Geometry check sheet. Reference: drawing and pictorial views, mm from the part's lowest x, y, z. Give positions to 0.01 mm unless a question says otherwise; leave off trailing zeros. Loops run counter-clockwise (first coordinate to the right, second up) from the corner with the lowest first, then second, coordinate; pieces in that order, holes last. Notation, with made-up numbers: (38, -39.5) - (43, -39.5) arc R32 cw to (43, -7.5) - close; hole circle Ø10 at (63, 19). An arc over 180 degrees is marked (long way). Use CSV: the item, a comma, the result in double quotes.
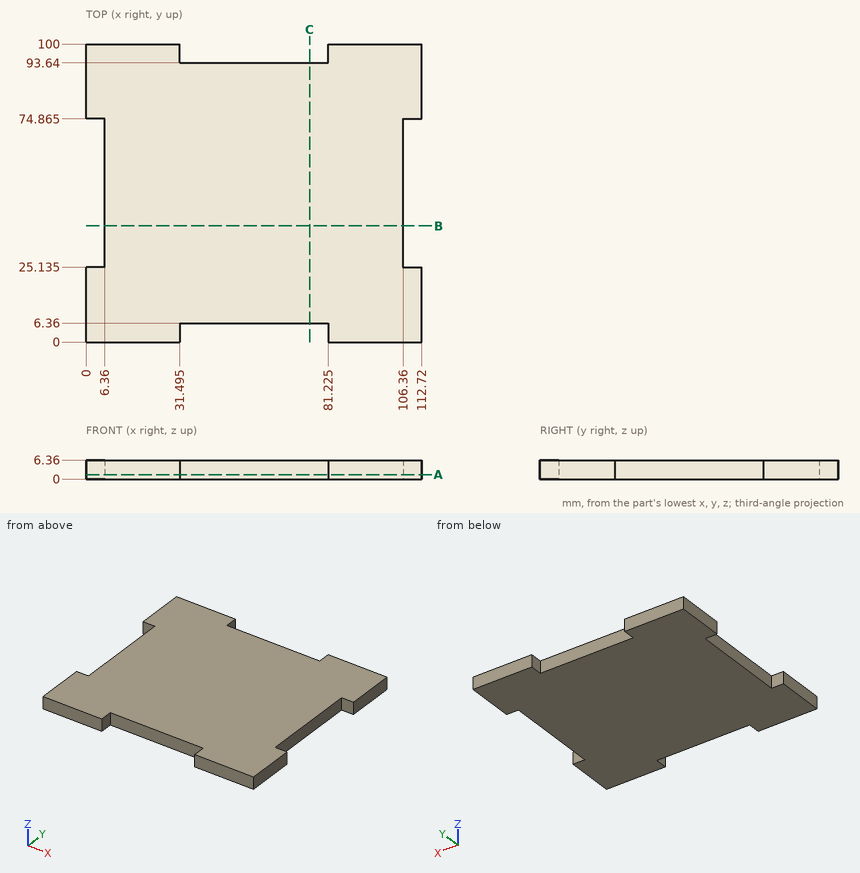
1. Go/stop test with flat-tipped pins: pin 1 Ø1.9 at (x, z) = (54, 2.5) entering from -Y; pin 2 Ø1.5 at (x, z) = (40.5, 5) entering from +Y; pin 3 Ø1.9 at (y, z) = (46.5, 2.5) entering from +X. Record where each tip stops, or that it passes through.
Completed:
pin 1,"stops at y = 6.36"
pin 2,"stops at y = 93.64"
pin 3,"stops at x = 106.36"
2. Sectioned sample at C-C, the plane x = 75. Record the boundary of the cut face in (y, z), and give its area (3 significant figures).
Completed:
outline,"(6.36, 0) - (93.64, 0) - (93.64, 6.36) - (6.36, 6.36) - close"
area,"555 mm²"
3. Sectioned sample at A-A, the plane z = 1.5. Record the boundary of the cut face in (x, y) (3 decimals).
Completed:
outline,"(0, 0) - (31.495, 0) - (31.495, 6.36) - (81.225, 6.36) - (81.225, 0) - (112.72, 0) - (112.72, 25.135) - (106.36, 25.135) - (106.36, 74.865) - (112.72, 74.865) - (112.72, 100) - (81.225, 100) - (81.225, 93.64) - (31.495, 93.64) - (31.495, 100) - (0, 100) - (0, 74.865) - (6.36, 74.865) - (6.36, 25.135) - (0, 25.135) - close"
4. Sectioned sample at B-B, the plane y = 39. Record the boundary of the cut face in (x, z).
Completed:
outline,"(6.36, 0) - (106.36, 0) - (106.36, 6.36) - (6.36, 6.36) - close"
5. Scan lines: line 1 along Y through (x, z) = (39, 4.75); line 2 along X through (y, z) = (29, 4.5). Record each from-to range of solid material in increasing order.
Completed:
line 1,"y = 6.36 to 93.64"
line 2,"x = 6.36 to 106.36"
